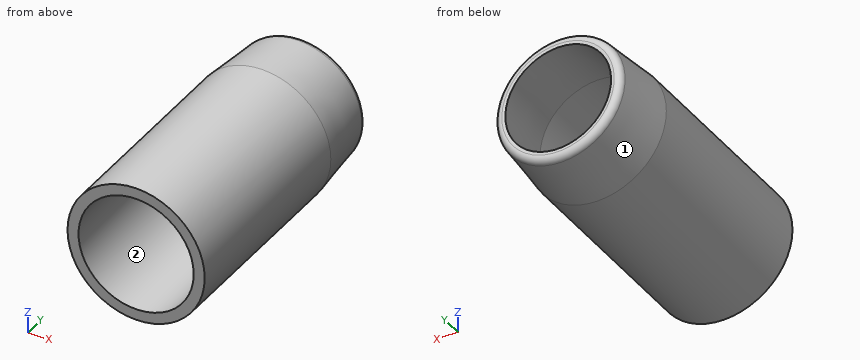
Autodesk Inventor part; units mm, degrees
ref_plane "Work Plane1" through (0, 0, 0) normal (1, 0, 0) x (0, 1, 0)
ref_plane "XZ Plane" through (0, 0, 0) normal (0, 1, 0) x (-1, 0, 0)
ref_plane "XY Plane" through (0, 0, 0) normal (0, 0, 1) x (1, 0, 0)
sketch "Sketch1" plane through (0, 0, 0) normal (0, 1, 0) x (-1, 0, 0)
  circle A0 centre (0, 0) radius 13.081
  dimension "d0" = 26.162
extrude "Extrusion1" add sketch "Sketch1" along normal blind 39.37
sketch "Sketch2" plane through (0, 39.37, 0) normal (0, 1, 0) x (1, 0, 0)
  circle A0 centre (0, 0) radius 10.9884
extrude "Extrusion2" cut sketch "Sketch2" against normal through all
sketch "Sketch3" plane through (0, 39.37, 0) normal (0, 1, 0) x (1, 0, 0)
  point P0 (0, 0)
ref_plane "Work Plane1" through (0, 0, 0) normal (1, 0, 0) x (0, 1, 0)
sketch "Sketch4" plane through (0, 0, 0) normal (1, 0, 0) x (0, 1, 0)
  line L0 (39.37, -13.081) -> (39.37, 13.081)
  line L1 (39.37, 13.081) -> (52.07, 13.081) construction
  line L2 (39.37, 0) -> (51.6373, 0)
  line L3 (39.37, 10.9884) -> (39.37, -10.9884)
  line L4 (39.37, 10.9884) -> (51.7114, 10.0843)
  line L5 (39.37, 13.081) -> (50.6127, 12.0974)
  line L6 (39.37, 13.081) -> (50.6556, 13.081) construction
  line L7 (51.7671, 10.7215) -> (51.7114, 10.0843)
  arc A0 (51.7671, 10.7215) -> (50.6127, 12.0974) centre (50.502, 10.8322) ccw
  point P0 (0, 0)
  dimension "d6" = 12.7
  dimension "d8" = 5
  dimension "d9" = 1.27
revolve "Revolution1" add sketch "Sketch4" angle 360 about axis through (0, 39.37, 0) along (0, 1, 0)
sketch "Sketch5" plane through (0, 0, 0) normal (1, 0, 0) x (0, 1, 0)
  line L0 (39.37, -13.081) -> (39.37, 13.081)
  line L1 (39.37, 10.9828) -> (51.7114, 10.0843)
  line L2 (51.7114, 10.0843) -> (39.37, 10.9884)
  point P0 (0, 0)
properties part number "cylinder part"
Part model, mm, in its own coordinate system. Face numbers are marked on the shaded views. Coordinates: 2 decimals unless noted, no trailing zeros. Write each loop counter-clockwise with the first axis right and the second up, starting at its lowest first coordinate (ties: lowest second). Pieces come first, ordered by that corner, then holes.
Item 1: Pin check, flat tips, straight feed: pin 1 (5 mm diameter, centred on x = -4.5, y = 11, fed in from +Z); pin 2 (10 mm diameter, centred on x = -0.5, y = 10.5, fed in from +Z); pin 3 (1 mm diameter, centred on x = 4.5, y = 6.5, fed in from -Z); pin 4 (2 mm diameter, centred on x = -8, y = 33, fed in from -Z). Stop position of each tip, or through.
Item 2: Mould opens along X. For the marked faces 1 and 2 say: released by +X, released by -X, zero draft, split by the parting line, or undercut.
Item 3: Probe line 1 (Z direction, x = 0, y = 20); line 2 (X direction, y = 45.5, z = 6). List the from-to ranges inside material, lowest first.
Item 4: Slice it at B-B (y = 18). Write the cut outline in (x, z), and give its area (3 significant figures).
Item 5: Slice it at C-C (x = 0). Write the cut outline in (y, z).
Item 6: Slice it at A-A (z = 0). Write the cut outline in (x, y), and give its area (3 significant figures).
Item 7: Slice it at D-D (y = 44). Write the cut outline in (x, z), and give its area (3 significant figures).
Results found:
1. pin 1: stops at z = 12.93
1. pin 2: stops at z = 13.08
1. pin 3: stops at z = -12.45
1. pin 4: stops at z = -11.05
2. face 1: split by the parting line
2. face 2: undercut
3. line 1: z = -13.08 to -10.99, 10.99 to 13.08
3. line 2: x = -11.02 to -8.66, 8.66 to 11.02
4. outline: circle Ø26.16 at (0, 0); hole circle Ø21.98 at (0, 0)
4. area: 158 mm2
5. outline: (0, -13.08) - (39.37, -13.08) - (50.61, -12.1) arc R1.27 ccw to (51.77, -10.72) - (51.71, -10.08) - (39.37, -10.99) - (0, -10.99) - close; (0, 10.99) - (39.37, 10.99) - (51.71, 10.08) - (51.77, 10.72) arc R1.27 ccw to (50.61, 12.1) - (39.37, 13.08) - (0, 13.08) - close
6. outline: (-13.08, 0) - (-10.99, 0) - (-10.99, 39.37) - (-10.08, 51.71) - (-10.72, 51.77) arc R1.27 ccw to (-12.1, 50.61) - (-13.08, 39.37) - close; (10.08, 51.71) - (10.99, 39.37) - (10.99, 0) - (13.08, 0) - (13.08, 39.37) - (12.1, 50.61) arc R1.27 ccw to (10.72, 51.77) - close
6. area: 214 mm2
7. outline: circle Ø25.35 at (0, 0); hole circle Ø21.3 at (0, 0)
7. area: 149 mm2
